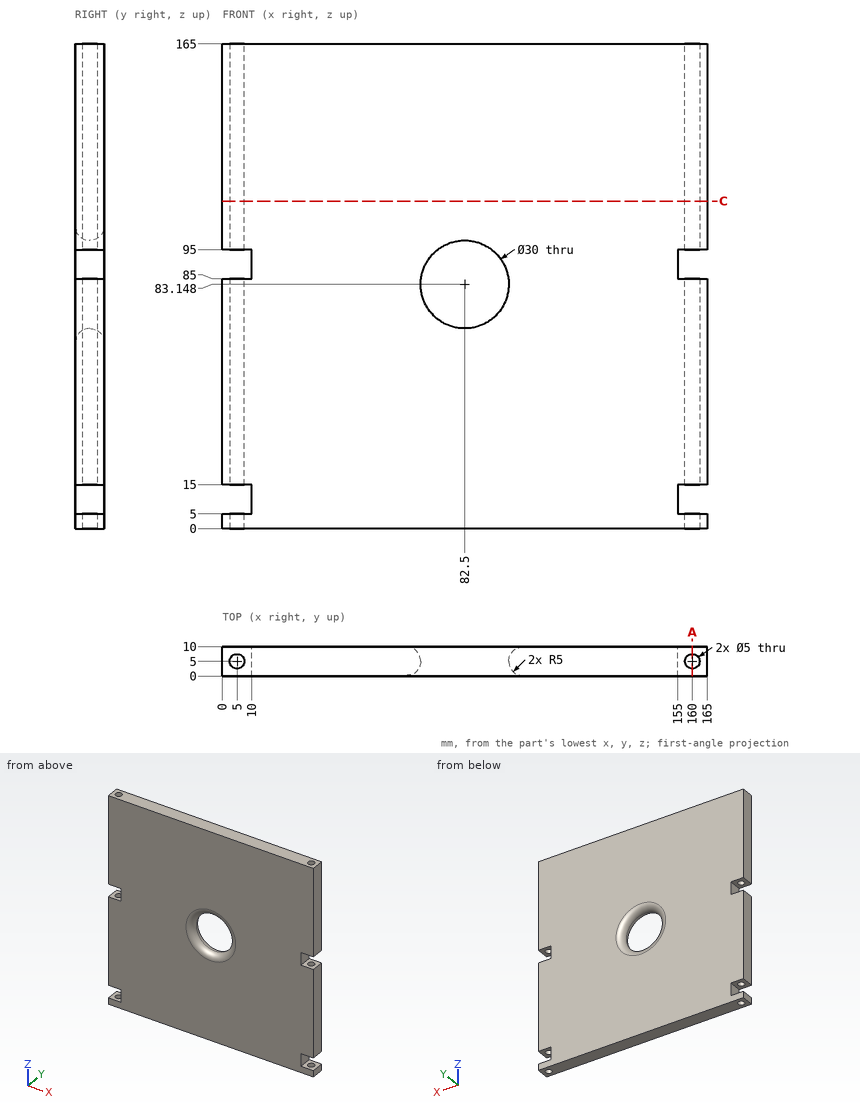
Verification items for this drawing (mm, ordinates from the low corner). Give positions to 0.01 mm unless a question says otherwise; leave off trailing zeros. Loops run counter-clockwise (first coordinate to the right, second up) from the corner with the lowest first, then second, coordinate; pieces in that order, holes last. Notation, with made-up numbers: M 69.25,62 L 102.25,62 A25 ccw 102.25,91 Z; hole C 1.25,-13 d4. An arc over 180 degrees is marked long. Answer as CSV lines item,"result".
Item 1: Material ranges on line 1 (Z direction, x = 156.5, y = 6); line 2 (Z direction, x = 82.5, y = 5.05); line 3 (X direction, y = 6.25, z = 122) (1 decimal), recorded low to high.
Values:
line 1,"z = 0 to 5, 15 to 85, 95 to 165"
line 2,"z = 0 to 68.15, 98.15 to 165"
line 3,"x = 0 to 2.8, 7.2 to 157.8, 162.2 to 165"
Item 2: Depth check by flat-ended pin: P1, Ø3, axis at y = 5.5, z = 88, coming from the +X side; P2, Ø3, axis at y = 5, z = 8.5, coming from the -X side. Enter the tip coordinate at first touch or a pass-through.
Values:
P1,"stops at x = 155"
P2,"stops at x = 10"
Item 3: Cross-section at A-A on x = 160. Record the cut outline in (y, z).
Values:
outline,"M 0,0 L 2.5,0 L 2.5,5 L 0,5 Z; M 0,15 L 2.5,15 L 2.5,85 L 0,85 Z; M 0,95 L 2.5,95 L 2.5,165 L 0,165 Z; M 7.5,0 L 10,0 L 10,5 L 7.5,5 Z; M 7.5,15 L 10,15 L 10,85 L 7.5,85 Z; M 7.5,95 L 10,95 L 10,165 L 7.5,165 Z"
Item 4: Cross-section at C-C on z = 111.5. Record the cut outline in (x, y).
Values:
outline,"M 0,0 L 165,0 L 165,10 L 0,10 Z; hole C 5,5 d5; hole C 160,5 d5"
